Here's how the part is built. I have some questions about the finished solid (model axes, mm). Face numbers are marked on the shaded views. A direction names the side the tool comes from. Coordinates: 2 decimals unless noted, no trailing zeros. Write each loop counter-clockwise with the first axis right and the second up, starting at its lowest first coordinate (ties: lowest second). Pieces come first, ordered by that corner, then holes. Notation, with made-up numbers: (3.5, 45.25) -> (47.5, 45.25) arc R26 ccw to (47.5, 60.25) -> close; hole circle Ø9 at (81, 38). An arc over 180 degrees is marked (long way). Put each result on its own line as item: value. Start each with the question number.
Item 1: I want a section at B-B, the plane x = 0. List the corners of the cut face in (y, z) for me, then the cut area to 3 significant figures.
Item 2: On a 3-axis mill with a long thin cutter (end or side, diameter ignored), from which of +Z, -Z, +X, -X, +Y, -Y can I reach the whole of each face in a straight line? I mean the marked faces 5, 6 and 7. Say none if no direction works.
Item 3: I want a section at A-A, the plane z = 0. List the corners of the cut face in (x, y) for me.
Item 4: I need wall thicknesses on line 1 (X direction, y = 4, z = 0); line 2 (X direction, y = 4.4, z = -0.5); line 3 (Y direction, x = -1, z = 0.5). Which ranges of each line are inside material? Lowest first, please. Write a range as [from, to].
Item 5: I want a section at D-D, the plane z = -4.25. List the corners of the cut face in (x, y) for me.
Item 6: I want a section at C-C, the plane y = 2.7. List the corners of the cut face in (x, z) for me, then the cut area to 3 significant figures.
Item 7: For pin 1 (1 mm diameter, centred on y = 4, z = 2.5, fed in from -X); pin 2 (1 mm diameter, centred on x = 0, z = -0.5, fed in from +Y); pin 3 (1 mm diameter, centred on x = 3, y = 4, fed in from -Z); pin 4 (3.5 mm diameter, centred on x = 0, z = 0, fed in from +Y), each with a flat end and sliding along its axis, tell me the tip position at first contact or that it passes through.
Item 8: If we mould it in two halves opening along Z, with no side actions, what happens to the marked faces 1, 2, 3 and 4? For each: released by +Z, released by -Z, zero draft, split by the parting line, or undercut.
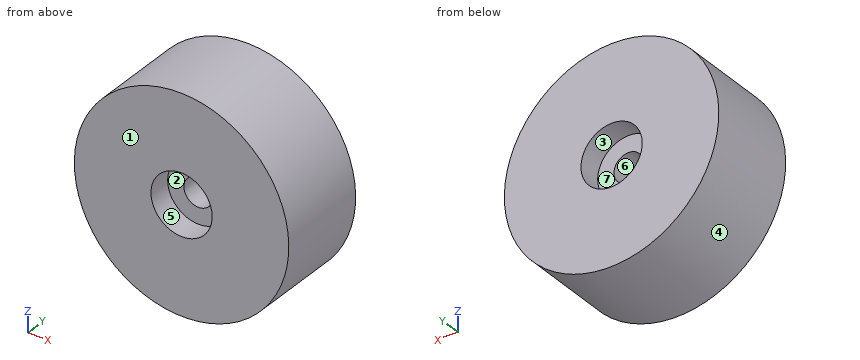
from build123d import *

# Parameters (mm, degrees)
SKETCH_1_R          = 5.6
EXTRUDE_1_DEPTH     = 4.8
SKETCH_2_R          = 0.75
CUT_EXTRUDE_1_DEPTH = 10.260669522
SKETCH_2_3_R        = 1.6
CUT_EXTRUDE_2_DEPTH = 1.2
CUT_EXTRUDE_START   = -3.6
SKETCH_2_4_R        = 1.6
CUT_EXTRUDE_3_DEPTH = 1.2


with BuildPart() as part:
    # 草图1 → 凸台-拉伸1 (new body)
    with BuildSketch(Plane(origin=(0, 0, 0), x_dir=(1, 0, 0), z_dir=(0, 1, 0))):
        with Locations(Location((0, 0, 0), (0, 0, 270))):
            Circle(SKETCH_1_R)
    extrude(amount=EXTRUDE_1_DEPTH)

    # 草图2 → 切除-拉伸1 (cut, through all)
    with BuildSketch(Plane(origin=(0, 4.8, 0), x_dir=(1, 0, 0), z_dir=(0, 1, 0))):
        with Locations(Location((0, 0, 0), (0, 0, 270))):
            Circle(SKETCH_2_R)
    extrude(amount=-CUT_EXTRUDE_1_DEPTH, mode=Mode.SUBTRACT)

    # 草图2<3> → 切除-拉伸2 (cut)
    with BuildSketch(Plane(origin=(0, 4.8, 0), x_dir=(1, 0, 0), z_dir=(0, 1, 0))):
        with Locations(Location((0, 0, 0), (0, 0, 270))):
            Circle(SKETCH_2_3_R)
    extrude(amount=-CUT_EXTRUDE_2_DEPTH, mode=Mode.SUBTRACT)

    # 草图2<4> → 切除-拉伸3 (cut)
    with BuildSketch(Plane(origin=(0, 4.8, 0), x_dir=(1, 0, 0), z_dir=(0, 1, 0)).offset(CUT_EXTRUDE_START)):
        with Locations(Location((0, 0, 0), (0, 0, 270))):
            Circle(SKETCH_2_4_R)
    extrude(amount=-CUT_EXTRUDE_3_DEPTH, mode=Mode.SUBTRACT)


solid = part.part
Calculated:
1. outline: (0, -5.6) -> (4.8, -5.6) -> (4.8, -1.6) -> (3.6, -1.6) -> (3.6, -0.75) -> (1.2, -0.75) -> (1.2, -1.6) -> (0, -1.6) -> close; (0, 1.6) -> (1.2, 1.6) -> (1.2, 0.75) -> (3.6, 0.75) -> (3.6, 1.6) -> (4.8, 1.6) -> (4.8, 5.6) -> (0, 5.6) -> close
1. area: 42.5 mm2
2. face 5: -Y
2. face 6: +Y, -Y
2. face 7: +Y
3. outline: (-5.6, 0) -> (-1.6, 0) -> (-1.6, 1.2) -> (-0.75, 1.2) -> (-0.75, 3.6) -> (-1.6, 3.6) -> (-1.6, 4.8) -> (-5.6, 4.8) -> close; (0.75, 1.2) -> (1.6, 1.2) -> (1.6, 0) -> (5.6, 0) -> (5.6, 4.8) -> (1.6, 4.8) -> (1.6, 3.6) -> (0.75, 3.6) -> close
4. line 1: x = [-5.6, -1.6], [1.6, 5.6]
4. line 2: x = [-5.58, -1.52], [1.52, 5.58]
4. line 3: y = [1.2, 3.6]
5. outline: (-3.65, 0) -> (3.65, 0) -> (3.65, 4.8) -> (-3.65, 4.8) -> close
6. outline: circle Ø11.2 at (0, 0); hole circle Ø1.5 at (0, 0)
6. area: 96.8 mm2
7. pin 1: stops at x = -5.23
7. pin 2: stops at y = 3.6
7. pin 3: stops at z = -5.01
7. pin 4: stops at y = 4.8
8. face 1: zero draft
8. face 2: undercut
8. face 3: undercut
8. face 4: split by the parting line
